```python
from build123d import *

# Parameters (mm, degrees)
SKETCH1_R           = 4
SKETCH1_W           = 9
SKETCH1_H           = 26.666666667
BOSS_EXTRUDE1_DEPTH = 9


with BuildPart() as part:
    # Sketch1 → Boss-Extrude1 (new body)
    # profile 1 of 5: a face of its own
    with BuildSketch(Plane(origin=(0, 0, 0), x_dir=(1, 0, 0), z_dir=(0, 1, 0))):
        Polygon((9, 26.666666667), (9, 0), (221, 0), (221, 26.666666667), (221, 53.333333333), (221, 80), (9, 80), (9, 53.333333333), align=None)
        with Locations(Location((67.5, 40, 0), (0, 0, 270))):
            Circle(SKETCH1_R, mode=Mode.SUBTRACT)
        with Locations(Location((162.5, 40, 0), (0, 0, 270))):
            Circle(SKETCH1_R, mode=Mode.SUBTRACT)
    # profile 2 of 5: a face of its own
    with BuildSketch(Plane(origin=(0, 0, 0), x_dir=(1, 0, 0), z_dir=(0, 1, 0))):
        with Locations((4.5, 66.666666667)):
            Rectangle(SKETCH1_W, SKETCH1_H)
    # profile 3 of 5: a face of its own
    with BuildSketch(Plane(origin=(0, 0, 0), x_dir=(1, 0, 0), z_dir=(0, 1, 0))):
        with Locations((4.5, 13.333333334)):
            Rectangle(SKETCH1_W, SKETCH1_H)
    # profile 4 of 5: a face of its own
    with BuildSketch(Plane(origin=(0, 0, 0), x_dir=(1, 0, 0), z_dir=(0, 1, 0))):
        with Locations((225.5, 66.666666667)):
            Rectangle(SKETCH1_W, SKETCH1_H)
    # profile 5 of 5: a face of its own
    with BuildSketch(Plane(origin=(0, 0, 0), x_dir=(1, 0, 0), z_dir=(0, 1, 0))):
        with Locations((225.5, 13.333333334)):
            Rectangle(SKETCH1_W, SKETCH1_H)
    extrude(amount=BOSS_EXTRUDE1_DEPTH)


solid = part.part
```
The listing builds one solid part. Answer for the finished solid, in the listing's coordinates (mm). A direction names the side the tool comes from. Coordinates: 2 decimals unless noted, no trailing zeros. Loops run counter-clockwise (first coordinate to the right, second up) from the corner with the lowest first, then second, coordinate; pieces in that order, holes last. Notation, with made-up numbers: (87.25, -38.5) - (106.25, -38.5) arc R18 ccw to (106.25, -21.5) - close; hole circle Ø10 at (13, 44). An arc over 180 degrees is marked (long way). Use a Markdown table: item, result. Add a question column.
1) The part is cut by section A-A, the plane x = 67.5. Give the vertices of the cut face in (y, z).
2) For faces 1 (the flat face through (4, 4, -26.667)), 2 (the flat face through (225, 4, -53.333)), 3 (the cylindrical face through (63.595, 4.437, -40.867)), determine the directions among +Z, -Z, +X, -X, +Y, -Y from which every point of the face is accessible in a straight line to the end or side of a thin tool.
3) The part is cut by section D-D, the plane z = -49.5. Give the vertices of the cut face in (x, y).
4) The part is cut by section C-C, the plane y = 6.25. Give the vertices of the cut face in (x, z).
5) Given pin 1 (9 mm diameter, centred on x = 67.5, z = -40, fed in from +Y); pin 2 (4 mm diameter, centred on y = 7, z = -37, fed in from +X), each flat-ended and moving along its own axis, determine where each tip first touches the part or whether it passes through.
6) Find the intervals of material crossed by line 1 (X direction, y = 6.25, z = -40); line 2 (X direction, y = 6, z = -30.5); line 3 (Z direction, x = 165.5, y = 1.25), in increasing order.
7) The mould has two halves that part along Z. Classify faces 4 (the flat face through (113, 4, 0)), 5 (the flat face through (113, 0, -41)), 6 (the flat face through (221, 4, -40)): released by +Z, released by -Z, zero draft, split by the parting line, or undercut.
8) The part is cut by section B-B, the plane z = -40. Give the vertices of the cut face in (x, y), and give its area (3 significant figures).
Here are the results:
| question | item | result |
|---|---|---|
| 1 | outline | (0, -80) - (9, -80) - (9, -44) - (0, -44) - close; (0, -36) - (9, -36) - (9, 0) - (0, 0) - close |
| 2 | face 1 | -X, +Y, -Y |
| 2 | face 2 | +X, +Y, -Y |
| 2 | face 3 | +Y, -Y |
| 3 | outline | (9, 0) - (221, 0) - (221, 9) - (9, 9) - close |
| 4 | outline | (0, -80) - (230, -80) - (230, -53.33) - (221, -53.33) - (221, -26.67) - (230, -26.67) - (230, 0) - (0, 0) - (0, -26.67) - (9, -26.67) - (9, -53.33) - (0, -53.33) - close; hole circle Ø8 at (67.5, -40); hole circle Ø8 at (162.5, -40) |
| 5 | pin 1 | stops at y = 9 |
| 5 | pin 2 | stops at x = 221 |
| 6 | line 1 | x = 9 to 63.5, 71.5 to 158.5, 166.5 to 221 |
| 6 | line 2 | x = 9 to 221 |
| 6 | line 3 | z = -80 to -42.65, -37.35 to 0 |
| 7 | face 4 | released by +Z |
| 7 | face 5 | zero draft |
| 7 | face 6 | undercut |
| 8 | outline | (9, 0) - (63.5, 0) - (63.5, 9) - (9, 9) - close; (71.5, 0) - (158.5, 0) - (158.5, 9) - (71.5, 9) - close; (166.5, 0) - (221, 0) - (221, 9) - (166.5, 9) - close |
| 8 | area | 1,760 mm^2 |
